Input: dimensioned drawing with shaded views. Units: mm. Origin: part minimum x, y, z. A direction names the side the tool comes from. Round coordinates to 2 decimals unless told otherwise and drop trailing zeros. Order: outer loops, then holes, each group sorted by start corner. A loop starts at its lowest first (then second) coordinate and runs counter-clockwise, first axis right, second up. Notation, with made-up numbers: M -2,71 L 12,71 A7 ccw 12,82 Z; hole C -26.75,7 d11. An arc over 180 degrees is marked long. Put each result on its own line as item: value. Start each with the question number.
1) Material intervals for probe 1 along Z at (x, y) = (65, 23.5); probe 2 along Z at (x, y) = (75, 31.5); probe 3 along Y at (x, z) = (49, 176.5) (1 decimal), sorted ascending. Write a range as [from, to].
2) First-contact query: P1, Ø1, axis at x = 38.5, y = 64, coming from the +Z side; P2, Ø13, axis at x = 37.5, y = 33, coming from the +Z side; P3, Ø8, axis at x = 56.5, z = 156.5, coming from the +Y side (1 decimal). Flat tips, straight axial feed; report the tip coordinate or a pass-through.
3) Section C-C, the plane z = 173.5. Return loops of the section in (x, y), then the cut area to 3 significant figures.
4) Section A-A, the plane x = 19.5. Return loops of the section in (y, z) (1 decimal), then the cut area to 3 significant figures.
5) Access query for the marked faces 1 and 2. Directions: +Z, -Z, +X, -X, +Y, -Y. A direction counts if a zero-diameter tool reaches every point of the face in a straight line with its end or side. Return the directions, or none.
6) Section B-B, the plane y = 29. Return loops of the section in (x, z).
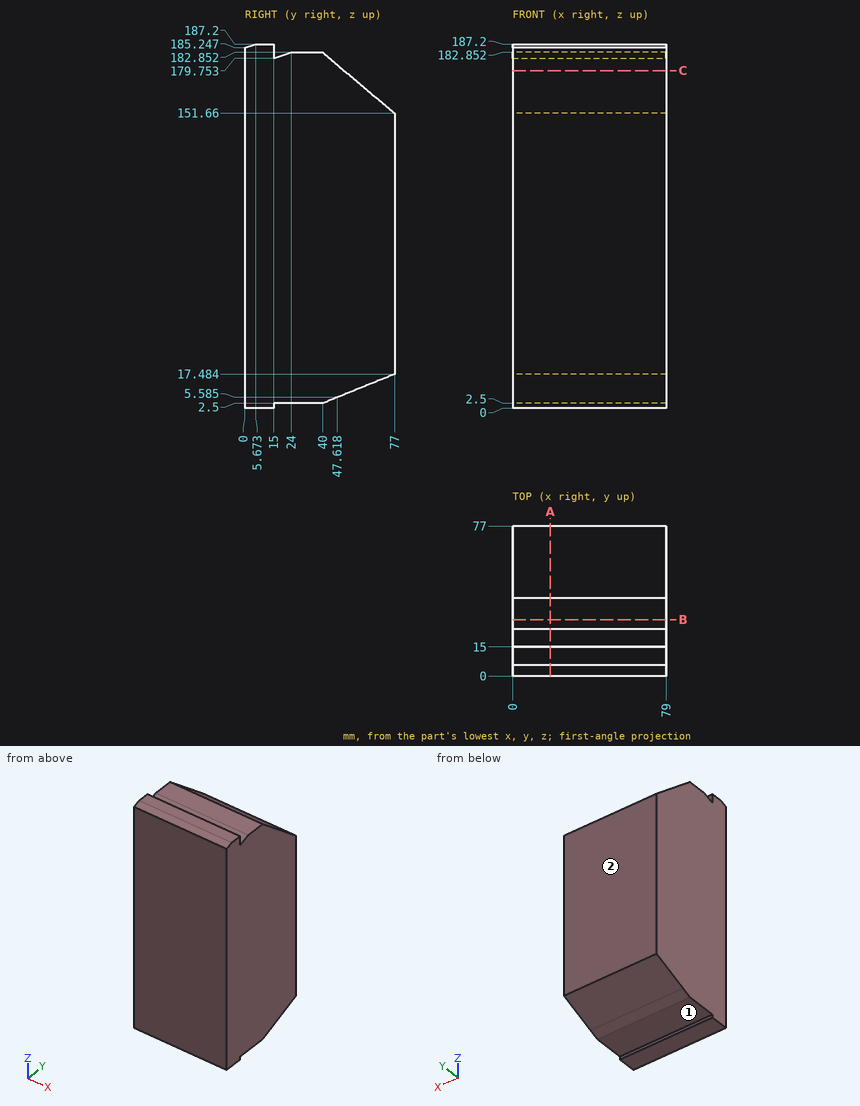
Result sheet:
1. probe 1: z = [2.5, 182.68]
1. probe 2: z = [2.5, 182.85]
1. probe 3: y = [0, 47.5]
2. P1: stops at z = 163.04
2. P2: stops at z = 182.85
2. P3: stops at y = 76
3. outline: M 0,0 L 79,0 L 79,51.09 L 0,51.09 Z
3. area: 4,040 mm2
4. outline: M 0,0 L 15,0 L 15,2.5 L 40,2.5 L 77,17.5 L 77,151.7 L 40,182.9 L 24,182.9 L 15,179.8 L 15,187.2 L 5.7,187.2 L 0,185.2 Z
4. area: 13,100 mm2
5. face 1: -Z, +X, -X, +Y
5. face 2: +Z, -Z, +X, -X, +Y
6. outline: M 0,2.5 L 79,2.5 L 79,182.85 L 0,182.85 Z
